For this review, take the finished solid that the model builds, in its own axes (mm). A direction names the side the tool comes from. Coordinates: 2 decimals unless noted, no trailing zeros. Write each loop counter-clockwise with the first axis right and the second up, starting at its lowest first coordinate (ties: lowest second). Pieces come first, ordered by that corner, then holes. Notation, with made-up numbers: (63, -17.5) -> (121, -17.5) arc R29 ccw to (121, 6.5) -> close; hole circle Ø11 at (73.25, 51.25). An arc over 180 degrees is marked (long way). Put each result on its own line as item: value. Start each with the question number.
Item 1: Consider section C-C on z = 30. Give the boundary of the cut face in (x, y) (3 decimals).
Item 2: The part is to be moulded in two halves that separate along Y. For faces 4 (the cylindrical face through (-0.69, 3.1, 1.28)), 5 (the flat face through (0, 0, 0)), 6 (the flat face through (0, 0, 18.6)), say which applies: +Y half, -Y half, draft (parallel to the pull), parting line (faces both ways), or undercut.
Item 3: Insertion check: P1, Ø1, axis at x = 2.5, z = 23, coming from the +Y side. The pin has a flat end and moves straight along its axis. Give the tip position at first contact, or say it passes through.
Item 4: To check wall thickness, follow L1, parallel to Y at x = 0, z = 28.75 (3 decimals); L2, parallel to Z at x = -2, y = 2. State the ranges of each line that lie inside material, in increasing order.
Item 5: For faces 1 (the cylindrical face through (1.5, -0.07, 26.2)), 2 (the cylindrical face through (0.69, -3.1, 23.46)), 3 (the flat face through (-0.8, -2.1, 2.6)), list the 3-axis set-ups (+Z, -Z, +X, -X, +Y, -Y) from which the entire face can be reached by the end or side of a thin tool; tool diameter is ignored.
Item 6: Consider section D-D on z = 4.5. Give the boundary of the cut face in (x, y).
Item 7: Consider section A-A on x = 0. Give the boundary of the cut face in (y, z) (1 decimal), and give its area (3 significant figures).
Autodesk Fusion 360 part; units mm, degrees
sketch "Sketch1" plane through (0, 0, 0) normal (0, 0, 1) x (1, 0, 0)
  circle A0 centre (0, 0) radius 3.175
  dimension "d1" = 6.35
extrude "Extrude1" add sketch "Sketch1" along normal blind 2.6
sketch "Sketch2" plane through (0, 0, 2.6) normal (0, 0, 1) x (-1, 0, 0)
  circle A0 centre (0, 0) radius 3.175
  circle A1 centre (0, 0) radius 2.0955
  dimension "d4" = 4.191
extrude "Extrude2" add sketch "Sketch2" along normal blind 11 contours A1
sketch "Sketch3" plane through (0, 0, 13.6) normal (0, 0, 1) x (-1, 0, 0)
  circle A0 centre (0, 0) radius 2.0955
  circle A1 centre (0, 0) radius 3.175
  dimension "d7" = 6.35
extrude "Extrude3" add sketch "Sketch3" along normal blind 20 contours A0 | A1
sketch "Sketch4" plane through (0, 0, 33.6) normal (0, 0, 1) x (-1, 0, 0)
  circle A0 centre (0, 0) radius 3.175
  circle A1 centre (0, 0) radius 1.5
  dimension "d10" = 3
extrude "Extrude4" cut sketch "Sketch4" against normal blind 15 contours A1
Return value:
1. outline: circle Ø6.35 at (0, 0); hole circle Ø3 at (0, 0)
2. face 4: parting line
2. face 5: draft
2. face 6: undercut
3. P1: y = 2.47
4. L1: -3.175 to -1.5, 1.5 to 3.175
4. L2: 0 to 2.6, 13.6 to 33.6
5. face 1: +Z
5. face 2: +Z, -Z
5. face 3: none
6. outline: circle Ø4.19 at (0, 0)
7. outline: (-3.2, 0) -> (3.2, 0) -> (3.2, 2.6) -> (2.1, 2.6) -> (2.1, 13.6) -> (3.2, 13.6) -> (3.2, 33.6) -> (1.5, 33.6) -> (1.5, 18.6) -> (-1.5, 18.6) -> (-1.5, 33.6) -> (-3.2, 33.6) -> (-3.2, 13.6) -> (-2.1, 13.6) -> (-2.1, 2.6) -> (-3.2, 2.6) -> close
7. area: 145 mm^2
